The listing builds one solid part. Answer for the finished solid, in the listing's coordinates (mm). Round coordinates to 2 decimals unless told otherwise and drop trailing zeros. Write each loop counter-clockwise with the first axis right and the second up, starting at its lowest first coordinate (ties: lowest second). Pieces come first, ordered by that corner, then holes. Notation, with made-up numbers: (81.25, 67) -> (140.25, 67) arc R30 ccw to (140.25, 104) -> close; hole circle Ø11 at (-26.75, 2). An arc over 180 degrees is marked (long way). Write each question's results on one line, items separated by ' | '. Start each with the question number.
```python
from build123d import *

# Parameters (mm, degrees)
BOSS_EXTRUDE1_DEPTH = 1000.125
CUT_EXTRUDE1_DEPTH  = 1001.125


with BuildPart() as part:
    # Sketch1 → Boss-Extrude1 (new body)
    with BuildSketch(Plane.XY):
        with BuildLine():
            Line((1.524, 0), (17.526, 0))
            ThreePointArc((17.526, 0), (18.603630735, 0.446369265), (19.05, 1.524))
            Line((19.05, 1.524), (19.05, 17.526))
            ThreePointArc((19.05, 17.526), (18.603630735, 18.603630735), (17.526, 19.05))
            Line((17.526, 19.05), (1.524, 19.05))
            ThreePointArc((1.524, 19.05), (0.446369265, 18.603630735), (0, 17.526))
            Line((0, 17.526), (0, 1.524))
            ThreePointArc((0, 1.524), (0.446369265, 0.446369265), (1.524, 0))
        make_face()
    extrude(amount=-BOSS_EXTRUDE1_DEPTH)

    # Sketch2 → Cut-Extrude1 (cut, through all)
    with BuildSketch(Plane.XY):
        with BuildLine():
            Line((5.08, 17.145), (13.97, 17.145))
            ThreePointArc((13.97, 17.145), (16.21506403, 16.21506403), (17.145, 13.97))
            Line((17.145, 13.97), (17.145, 5.08))
            ThreePointArc((17.145, 5.08), (16.21506403, 2.83493597), (13.97, 1.905))
            Line((13.97, 1.905), (5.08, 1.905))
            ThreePointArc((5.08, 1.905), (2.83493597, 2.83493597), (1.905, 5.08))
            Line((1.905, 5.08), (1.905, 13.97))
            ThreePointArc((1.905, 13.97), (2.83493597, 16.21506403), (5.08, 17.145))
        make_face()
    extrude(amount=-CUT_EXTRUDE1_DEPTH, mode=Mode.SUBTRACT)


solid = part.part
```
Q1. The part is cut by section A-A, the plane x = 9.5. Write down the section's boundary in (y, z) (3 decimals).
Q2. This flat-tipped pin is pushed along its axis until it touches: pin 1 (1 mm diameter, centred on x = 11, y = 15.5, fed in from +Z). Where does it stop, or does it pass through?
Q3. The part is cut by section B-B, the plane z = -938. Write down the section's boundary in (x, y) (3 decimals), then the cut area to 3 significant figures.
Q4. Find the intervals of material crossed by line 1 (X direction, y = 9.75, z = -492) (3 decimals); line 2 (Y direction, x = 15, z = -101), in increasing order.
Answers follow:
1) outline: (0, -1000.125) -> (1.905, -1000.125) -> (1.905, 0) -> (0, 0) -> close; (17.145, -1000.125) -> (19.05, -1000.125) -> (19.05, 0) -> (17.145, 0) -> close
2) pin 1: through
3) outline: (0, 1.524) arc R1.524 ccw to (1.524, 0) -> (17.526, 0) arc R1.524 ccw to (19.05, 1.524) -> (19.05, 17.526) arc R1.524 ccw to (17.526, 19.05) -> (1.524, 19.05) arc R1.524 ccw to (0, 17.526) -> close; hole (1.905, 5.08) arc R3.175 ccw to (5.08, 1.905) -> (13.97, 1.905) arc R3.175 ccw to (17.145, 5.08) -> (17.145, 13.97) arc R3.175 ccw to (13.97, 17.145) -> (5.08, 17.145) arc R3.175 ccw to (1.905, 13.97) -> close | area: 137 mm^2
4) line 1: 0 to 1.905, 17.145 to 19.05 | line 2: 0 to 2.08, 16.97 to 19.05
